from build123d import *

# Parameters (mm, degrees)
F0_R      = 3.175
F0_R_2    = 2.38125
F1_DEPTH  = 7.9375
F2_DEPTH  = 15.875
F3_W      = 3.175
F3_H      = 5.499262
F5_W      = 3.175
F5_H      = 4.7625
F7_R      = 1.5875
F8_DEPTH  = 0.79375
F9_R      = 1.5875
F10_DEPTH = 0.79375


with BuildPart() as f1:
    # F0 (on Front) → F1 (new body)
    with BuildSketch(Plane.XZ):
        Circle(F0_R)
        Circle(F0_R_2, mode=Mode.SUBTRACT)
    extrude(amount=F1_DEPTH)

    # F0 (on Front) → F2 (join)
    with BuildSketch(Plane.XZ):
        Circle(F0_R_2)
    extrude(amount=F2_DEPTH)

    # F3 (on face) → F6 section 0
    with BuildSketch(Plane(origin=(0, 0, 0), x_dir=(-1, 0, 0), z_dir=(0, 1, 0))):
        Rectangle(F3_W, F3_H)
    # F5 (on offset) → F6 section 1
    with BuildSketch(Plane(origin=(0, 6.35, 0), x_dir=(-1, 0, 0), z_dir=(0, 1, 0))):
        Rectangle(F5_W, F5_H)
    loft()

    # F7 (on face) → F8 (cut)
    with BuildSketch(Plane.YZ.offset(1.5875)):
        with Locations((3.175, 0)):
            Circle(F7_R)
    extrude(amount=-F8_DEPTH, mode=Mode.SUBTRACT)

    # F9 (on face) → F10 (cut)
    with BuildSketch(Plane(origin=(-1.5875, 0, 0), x_dir=(0, -1, 0), z_dir=(-1, 0, 0))):
        with Locations((-3.175, 0)):
            Circle(F9_R)
    extrude(amount=-F10_DEPTH, mode=Mode.SUBTRACT)


solid = f1.part
Input: part model. Units: mm. Frame: model coordinates. A direction names the side the tool comes from. Give positions to 0.01 mm unless a question says otherwise; leave off trailing zeros. Order: outer loops, then holes, each group sorted by start corner. A loop starts at its lowest first (then second) coordinate and runs counter-clockwise, first axis right, second up.
Q1. Ray query, probe 1 along Y at (x, z) = (1.75, -0.75) (3 decimals); probe 2 along X at (y, z) = (5, 0); probe 3 along X at (y, z) = (-12.5, -1.25). Return the intervals inside material, ascending.
Checked values:
probe 1: y = -15.875 to 0
probe 2: x = -1.59 to 1.59
probe 3: x = -2.03 to 2.03
Q2. Section C-C on y = -10.5. Output: boundary loops of the cut face in (x, z).
Checked values:
outline: circle Ø4.76 at (0, 0)
Q3. Draft query along Z for faces 4 (the flat face through (2, 0, 0)), 5 (the flat face through (0.794, 3, 0)), 6 (the cylindrical face through (-1.89, -11.85, -1.45)). Return one class per face: +Z half, -Z half, draft (parallel to the pull), parting line (faces both ways), or undercut.
Checked values:
face 4: draft
face 5: undercut
face 6: parting line
Q4. Set-up query: faces 1 (the cylindrical face through (1.2, 1.59, 0.07)), 2 (the flat face through (-0.794, 3, 0)), 3 (the flat face through (-2, 0, 0)). Return all of +Z, -Z, +X, -X, +Y, -Y with unobstructed straight access to the full face (end or side cutting, diameter ignored); none if empty.
Checked values:
face 1: +X
face 2: -X
face 3: +Z, -Z, -X, +Y
Q5. Section B-B on y = -2. Output: boundary loops of the cut face in (x, z) (3 decimals).
Checked values:
outline: circle Ø6.35 at (0, 0)
Q6. Contact query for flat-ended pins moving along their axis: pin 1 Ø1.7 at (x, z) = (2.5, -1.5) entering from +Y; pin 2 Ø3 at (y, z) = (-3, 2) entering from +X; pin 3 Ø3 at (y, z) = (3.175, 0) entering from +X. Output: stop coordinate, or through.
Checked values:
pin 1: stops at y = 0
pin 2: stops at x = 3.14
pin 3: stops at x = 0.79
